Could you check a few things on this model? Use its own coordinates, in mm. A direction names the side the tool comes from. Round coordinates to 2 decimals unless told otherwise and drop trailing zeros. Loops run counter-clockwise (first coordinate to the right, second up) from the corner with the lowest first, then second, coordinate; pieces in that order, holes last. Notation, with made-up numbers: (80.5, 11) -> (125.5, 11) arc R17 cw to (125.5, 27) -> close; hole circle Ø3 at (-16.5, 42). An arc over 180 degrees is marked (long way). One line per item, written item: value.
```python
from build123d import *

# Parameters (mm, degrees)
BOSS_EXTRUDE1_DEPTH = 7.62


with BuildPart() as part:
    # Sketch1 → Boss-Extrude1 (new body)
    with BuildSketch(Plane.XY):
        with BuildLine():
            Line((73.084670889, 24.389207851), (79.434670889, 0.351172556))
            Line((79.434670889, 0.351172556), (104.834670889, 0.351172556))
            Line((104.834670889, 0.351172556), (104.834670889, -7.268827444))
            Line((104.834670889, -7.268827444), (79.434670889, -7.268827444))
            Line((79.434670889, -7.268827444), (70.374307571, -30.552841702))
            Line((70.374307571, -30.552841702), (64.024307571, -30.552841702))
            ThreePointArc((64.024307571, -30.552841702), (63.754976443, -29.466421477), (63.079810248, -28.573673602))
            Line((63.079810248, -28.573673602), (62.683021764, -28.224932994))
            ThreePointArc((62.683021764, -28.224932994), (62.247675801, -27.79943175), (61.859720198, -27.330317834))
            ThreePointArc((61.859720198, -27.330317834), (61.688197961, -27.049614145), (61.569433036, -26.742841702))
            ThreePointArc((61.569433036, -26.742841702), (61.63789275, -25.531251133), (62.446208329, -24.626118898))
            ThreePointArc((62.446208329, -24.626118898), (62.747108688, -24.493177507), (63.066880707, -24.415974562))
            ThreePointArc((63.066880707, -24.415974562), (63.672920376, -24.358586969), (64.281631273, -24.365548236))
            Line((64.281631273, -24.365548236), (64.80879995, -24.399523215))
            ThreePointArc((64.80879995, -24.399523215), (65.544016286, -24.349243284), (66.240331439, -24.107962657))
            ThreePointArc((66.240331439, -24.107962657), (66.370344576, -23.747689015), (66.498398241, -23.386714262))
            ThreePointArc((66.498398241, -23.386714262), (66.113206158, -22.758464159), (65.576773496, -22.253180941))
            Line((65.576773496, -22.253180941), (65.147713099, -21.945011687))
            ThreePointArc((65.147713099, -21.945011687), (64.672757031, -21.564230714), (64.240688336, -21.135402009))
            ThreePointArc((64.240688336, -21.135402009), (64.042478252, -20.872862103), (63.894216256, -20.579207851))
            ThreePointArc((63.894216256, -20.579207851), (63.843589674, -19.366741197), (64.55929452, -18.38673864))
            ThreePointArc((64.55929452, -18.38673864), (64.845715425, -18.224944005), (65.156380444, -18.116769674))
            ThreePointArc((65.156380444, -18.116769674), (65.753876898, -18.000256143), (66.360339009, -17.947519788))
            Line((66.360339009, -17.947519788), (66.888299355, -17.929659602))
            ThreePointArc((66.888299355, -17.929659602), (67.615047129, -17.80755798), (68.284359697, -17.499188365))
            ThreePointArc((68.284359697, -17.499188365), (68.378433792, -17.127906023), (68.470489131, -16.756118009))
            ThreePointArc((68.470489131, -16.756118009), (68.025572575, -16.168648528), (67.442196566, -15.718377982))
            Line((67.442196566, -15.718377982), (66.984996344, -15.45374792))
            ThreePointArc((66.984996344, -15.45374792), (66.475004257, -15.121354347), (66.002983527, -14.736940707))
            ThreePointArc((66.002983527, -14.736940707), (65.779994468, -14.495092989), (65.603663244, -14.21738498))
            ThreePointArc((65.603663244, -14.21738498), (65.43443793, -13.015718957), (66.050639412, -11.970284037))
            ThreePointArc((66.050639412, -11.970284037), (66.319822476, -11.781194329), (66.618388618, -11.643090391))
            ThreePointArc((66.618388618, -11.643090391), (67.20158764, -11.46857301), (67.799960404, -11.356646914))
            Line((67.799960404, -11.356646914), (68.323627873, -11.287123566))
            ThreePointArc((68.323627873, -11.287123566), (69.034908105, -11.094376158), (69.670772242, -10.721887324))
            ThreePointArc((69.670772242, -10.721887324), (69.728001312, -10.343171934), (69.783171782, -9.964151179))
            ThreePointArc((69.783171782, -9.964151179), (69.282815542, -9.423119973), (68.658114417, -9.032198451))
            Line((68.658114417, -9.032198451), (68.177177456, -8.813656114))
            ThreePointArc((68.177177456, -8.813656114), (67.637060853, -8.532851072), (67.129633907, -8.196554611))
            ThreePointArc((67.129633907, -8.196554611), (66.884013379, -7.977728206), (66.681311093, -7.718640919))
            ThreePointArc((66.681311093, -7.718640919), (66.395116777, -6.539348227), (66.90588054, -5.438549056))
            ThreePointArc((66.90588054, -5.438549056), (67.155233381, -5.223985312), (67.438825293, -5.057281783))
            ThreePointArc((67.438825293, -5.057281783), (68.002110358, -4.82644125), (68.586631118, -4.656403321))
            Line((68.586631118, -4.656403321), (69.100962504, -4.53588636))
            ThreePointArc((69.100962504, -4.53588636), (69.789925178, -4.274349429), (70.386217165, -3.841328646))
            ThreePointArc((70.386217165, -3.841328646), (70.406050062, -3.458827444), (70.42380434, -3.076224127))
            ThreePointArc((70.42380434, -3.076224127), (69.872827121, -2.586841621), (69.212817092, -2.259033911))
            Line((69.212817092, -2.259033911), (68.71277508, -2.08868398))
            ThreePointArc((68.71277508, -2.08868398), (68.147735579, -1.862171777), (67.609789215, -1.577231214))
            ThreePointArc((67.609789215, -1.577231214), (67.343902678, -1.383533539), (67.116781464, -1.145562126))
            ThreePointArc((67.116781464, -1.145562126), (66.716374355, 0), (67.116781464, 1.145562126))
            ThreePointArc((67.116781464, 1.145562126), (67.343902678, 1.383533539), (67.609789215, 1.577231214))
            ThreePointArc((67.609789215, 1.577231214), (68.147735579, 1.862171777), (68.71277508, 2.08868398))
            Line((68.71277508, 2.08868398), (69.212817092, 2.259033911))
            ThreePointArc((69.212817092, 2.259033911), (69.872827121, 2.586841621), (70.42380434, 3.076224127))
            ThreePointArc((70.42380434, 3.076224127), (70.406050062, 3.458827444), (70.386217165, 3.841328646))
            ThreePointArc((70.386217165, 3.841328646), (69.789925178, 4.274349429), (69.100962504, 4.53588636))
            Line((69.100962504, 4.53588636), (68.586631118, 4.656403321))
            ThreePointArc((68.586631118, 4.656403321), (68.002110358, 4.82644125), (67.438825293, 5.057281783))
            ThreePointArc((67.438825293, 5.057281783), (67.155233381, 5.223985312), (66.90588054, 5.438549056))
            ThreePointArc((66.90588054, 5.438549056), (66.395116777, 6.539348227), (66.681311093, 7.718640919))
            ThreePointArc((66.681311093, 7.718640919), (66.884013379, 7.977728206), (67.129633907, 8.196554611))
            ThreePointArc((67.129633907, 8.196554611), (67.637060853, 8.532851072), (68.177177456, 8.813656114))
            Line((68.177177456, 8.813656114), (68.658114417, 9.032198451))
            ThreePointArc((68.658114417, 9.032198451), (69.282815542, 9.423119973), (69.783171782, 9.964151179))
            ThreePointArc((69.783171782, 9.964151179), (69.728001312, 10.343171934), (69.670772242, 10.721887324))
            ThreePointArc((69.670772242, 10.721887324), (69.034908105, 11.094376158), (68.323627873, 11.287123566))
            Line((68.323627873, 11.287123566), (67.799960404, 11.356646914))
            ThreePointArc((67.799960404, 11.356646914), (67.20158764, 11.46857301), (66.618388618, 11.643090391))
            ThreePointArc((66.618388618, 11.643090391), (66.319822476, 11.781194329), (66.050639412, 11.970284037))
            ThreePointArc((66.050639412, 11.970284037), (65.43443793, 13.015718957), (65.603663244, 14.21738498))
            ThreePointArc((65.603663244, 14.21738498), (65.779994468, 14.495092989), (66.002983527, 14.736940707))
            ThreePointArc((66.002983527, 14.736940707), (66.475004257, 15.121354347), (66.984996344, 15.45374792))
            Line((66.984996344, 15.45374792), (67.442196566, 15.718377982))
            ThreePointArc((67.442196566, 15.718377982), (68.025572575, 16.168648528), (68.470489131, 16.756118009))
            ThreePointArc((68.470489131, 16.756118009), (68.378433792, 17.127906023), (68.284359697, 17.499188365))
            ThreePointArc((68.284359697, 17.499188365), (67.615047129, 17.80755798), (66.888299355, 17.929659602))
            Line((66.888299355, 17.929659602), (66.360339009, 17.947519788))
            ThreePointArc((66.360339009, 17.947519788), (65.753876898, 18.000256143), (65.156380444, 18.116769674))
            ThreePointArc((65.156380444, 18.116769674), (64.845715425, 18.224944005), (64.55929452, 18.38673864))
            ThreePointArc((64.55929452, 18.38673864), (63.843589674, 19.366741197), (63.894216256, 20.579207851))
            ThreePointArc((63.894216256, 20.579207851), (64.042478252, 20.872862103), (64.240688336, 21.135402009))
            ThreePointArc((64.240688336, 21.135402009), (64.672757031, 21.564230714), (65.147713099, 21.945011687))
            Line((65.147713099, 21.945011687), (65.576773496, 22.253180941))
            ThreePointArc((65.576773496, 22.253180941), (66.400832851, 23.188324819), (66.734670889, 24.389207851))
            Line((66.734670889, 24.389207851), (73.084670889, 24.389207851))
        make_face()
    extrude(amount=BOSS_EXTRUDE1_DEPTH)


solid = part.part
```
Item 1: If we section it at B-B on x = 72.5: List the corners of the cut face in (y, z) for me, plus the area to 3 significant figures.
Output:
outline: (-25.09, 0) -> (24.39, 0) -> (24.39, 7.62) -> (-25.09, 7.62) -> close
area: 377 mm²
Item 2: I need wall thicknesses on line 1 (Y direction, x = 88.5, z = 4); line 2 (X direction, y = 10.5, z = 2.5); line 3 (X direction, y = 9, z = 6.5). Which ranges of each line are inside material? Lowest first, please. Write a range as from..to.
Output:
line 1: y = -7.27..0.35
line 2: x = 69.7..76.75
line 3: x = 68.59..77.15
Item 3: For faces 5 (the face through (69.8, 4.27, 3.76)), 6 (the face through (92, 0.351, 4)), 7 (the face through (66.39, 23.17, 3.76)), which set-ups out of +Z, -Z, +X, -X, +Y, -Y let a thin tool reach every point of the face, with its end or its side?
Output:
face 5: +Z, -Z, -X
face 6: +Z, -Z, +X, +Y
face 7: +Z, -Z, -X, +Y
Item 4: If we section it at A-A on x = 96.5: List the corners of the cut face in (y, z) for me.
Output:
outline: (-7.27, 0) -> (0.35, 0) -> (0.35, 7.62) -> (-7.27, 7.62) -> close
Item 5: If we mould it in two halves opening along X, with no side actions, what happens to faces 1 (the face through (92, -7.269, 4)), 2 (the face through (65.534, -24.351, 3.757)), 3 (the face through (69.88, -2.59, 3.76)), 4 (the face through (76.215, 12.538, 3.757))? For each: released by +X, released by -X, zero draft, split by the parting line, or undercut.
Output:
face 1: zero draft
face 2: undercut
face 3: released by -X
face 4: released by +X
Item 6: Will these pins go through, and if not, where does the flat tip stop? pin 1 Ø3 at (x, z) = (95, 1.5) entering from -Y; pin 2 Ø2 at (y, z) = (-16.5, 1.5) entering from -X; pin 3 Ø4 at (x, z) = (89.5, 3) entering from +Y.
Output:
pin 1: stops at y = -7.27
pin 2: stops at x = 67.06
pin 3: stops at y = 0.35
